Geometry check sheet. Reference: drawing and pictorial views, mm from the part's lowest x, y, z. A direction names the side the tool comes from. Coordinates: 2 decimals unless noted, no trailing zeros. Loops run counter-clockwise (first coordinate to the right, second up) from the corner with the lowest first, then second, coordinate; pieces in that order, holes last. Notation, with made-up numbers: (-10, 9.5) - (1, 9.5) arc R25 cw to (1, 32.5) - close; hole circle Ø7 at (-5, 69.25). An arc over 180 degrees is marked (long way). Write each question's results on one line, items separated by ' | '. Start each with the question number.
1. Cross-section at B-B (y = 15.5). Record the cut outline in (x, z).
2. Thickness scan on line 1 (Z direction, x = 16, y = 10.5); line 2 (X direction, y = 7.75, z = 5.5); line 3 (Y direction, x = 18.5, z = 9). Record the ranges inside material, lowest first. Write a range as [from, to].
3. Tool access check on the marked faces 1, 2 and 3. Record the directions out of +Z, -Z, +X, -X, +Y, -Y that give a thin tool (end or side, any length) a straight path to the whole face; none if there is none.
4. Cross-section at D-D (x = 33.6). Record the cut outline in (y, z).
5. Draft check along Z on the marked faces 4, 5 and 6. Enter one of: released by +Z, released by -Z, zero draft, split by the parting line, or undercut.
6. Gauge pin test, flat ends, axial feed: P1, Ø10, axis at x = 36.5, y = 17.5, coming from the -Z side; P2, Ø10, axis at x = 13.5, z = 35.5, coming from the +Y side; P3, Ø1.5, axis at x = 26, z = 41, coming from the +Y side; P4, Ø1.6, axis at y = 22.5, z = 44, coming from the +X side. Record the tip position at first contact, or that the pin passes through.
7. Cross-section at C-C (x = 15). Record the cut outline in (y, z), and give its area (3 significant figures).
8. Cross-section at A-A (z = 5.5). Record the cut outline in (x, y).
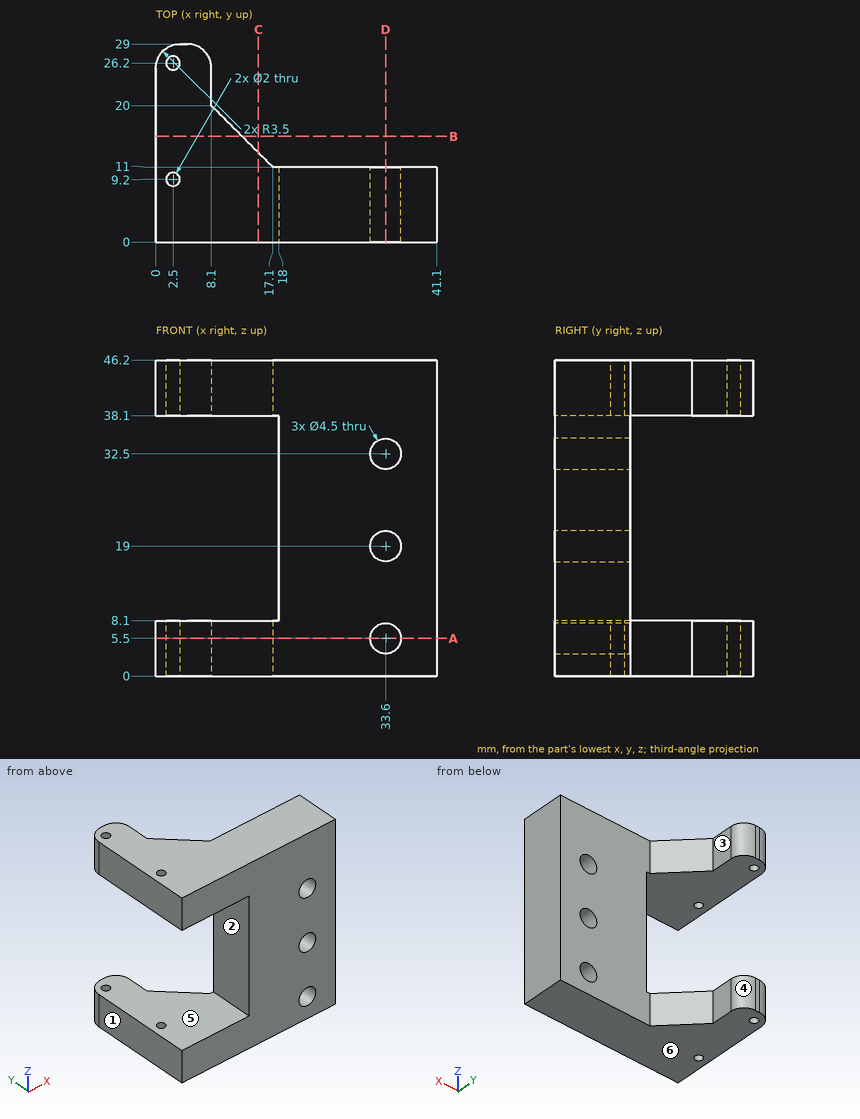
Established:
1) outline: (0, 0) - (12.6, 0) - (12.6, 8.1) - (0, 8.1) - close; (0, 38.1) - (12.6, 38.1) - (12.6, 46.2) - (0, 46.2) - close
2) line 1: [0, 8.1], [38.1, 46.2] | line 2: [0, 31.35], [35.85, 41.1] | line 3: [0, 11]
3) face 1: +Z, -Z, -X, +Y, -Y | face 2: -X, +Y, -Y | face 3: +Z, -Z, +X, +Y
4) outline: (0, 0) - (11, 0) - (11, 3.25) - (0, 3.25) - close; (0, 7.75) - (11, 7.75) - (11, 16.75) - (0, 16.75) - close; (0, 21.25) - (11, 21.25) - (11, 30.25) - (0, 30.25) - close; (0, 34.75) - (11, 34.75) - (11, 46.2) - (0, 46.2) - close
5) face 4: zero draft | face 5: undercut | face 6: released by -Z
6) P1: through | P2: y = 18.87 | P3: y = 11 | P4: x = 8.1
7) outline: (0, 0) - (13.1, 0) - (13.1, 8.1) - (0, 8.1) - close; (0, 38.1) - (13.1, 38.1) - (13.1, 46.2) - (0, 46.2) - close | area: 212 mm^2
8) outline: (0, 0) - (31.35, 0) - (31.35, 11) - (17.1, 11) - (8.1, 20) - (8.1, 25.5) arc R3.5 ccw to (4.6, 29) - (3.5, 29) arc R3.5 ccw to (0, 25.5) - close; (35.85, 0) - (41.1, 0) - (41.1, 11) - (35.85, 11) - close; hole circle Ø2 at (2.5, 9.2); hole circle Ø2 at (2.5, 26.2)
